```python
from build123d import *

# Parameters (mm, degrees)
SKETCH1_W               = 175
SKETCH1_H               = 260
BOSS_EXTRUDE1_DEPTH     = 3
SKETCH4_W               = 8.7
SKETCH4_H               = 8.7
BOSS_EXTRUDE3_DEPTH     = 328
MIRROR5_COPY_1_SKETCH_W = 8.7
MIRROR5_COPY_1_SKETCH_H = 8.7
MIRROR5_COPY_1_DEPTH    = 328
SKETCH6_W               = 38
SKETCH6_H               = 39
SKETCH6_W_2             = 34
SKETCH6_H_2             = 35
EXTRUDE_THIN1_DEPTH     = 10
SKETCH7_W               = 5.74
SKETCH7_H               = 5.74
BOSS_EXTRUDE5_DEPTH     = 8.5
SKETCH9_R               = 10.5
SKETCH9_R_2             = 6.5
EXTRUDE_THIN2_DEPTH     = 18
CUT_EXTRUDE1_DEPTH      = 367.180283467
CUT_EXTRUDE1_DEPTH_BACK = 367.180283467
SKETCH10_R              = 2.5
SKETCH11_R              = 2.5
BOSS_EXTRUDE6_DEPTH     = 3
CUT_EXTRUDE2_DEPTH      = 1
MIRROR7_COPY_1_SKETCH_R = 2.5
MIRROR7_COPY_1_DEPTH    = 3
MIRROR7_COPY_2_DEPTH    = 1


with BuildPart() as part:
    # Sketch1 → Boss-Extrude1 (new body)
    with BuildSketch(Plane(origin=(0, 0, 0), x_dir=(1, 0, 0), z_dir=(0, 1, 0))):
        Rectangle(SKETCH1_W, SKETCH1_H)
    extrude(amount=BOSS_EXTRUDE1_DEPTH)

    # Sketch4 → Boss-Extrude3 (add)
    with BuildSketch(Plane.XZ):
        with Locations((81.15, -123.65)):
            Rectangle(SKETCH4_W, SKETCH4_H)
    boss_extrude3 = extrude(amount=BOSS_EXTRUDE3_DEPTH)

    # Mirror3: Boss-Extrude3 across plane
    add(boss_extrude3.mirror(Plane.XY))

    # Mirror5: Boss-Extrude3 across plane
    add(boss_extrude3.mirror(Plane(origin=(0, 0, 0), x_dir=(0, 0, 1), z_dir=(1, 0, 0))))

    # Mirror5 copy 1 sketch → Mirror5 copy 1 (add)
    with BuildSketch(Plane(origin=(0, 0, 0), x_dir=(-1, 0, 0), z_dir=(0, -1, 0))):
        with Locations((81.15, -123.65)):
            Rectangle(MIRROR5_COPY_1_SKETCH_W, MIRROR5_COPY_1_SKETCH_H)
    extrude(amount=MIRROR5_COPY_1_DEPTH)

    # Sketch6 → Extrude-Thin1 (add)
    with BuildSketch(Plane(origin=(0, 0, -130), x_dir=(-1, 0, 0), z_dir=(0, 0, -1))):
        with Locations((0, -19.5)):
            Rectangle(SKETCH6_W, SKETCH6_H)
        with Locations((0, -19.5)):
            Rectangle(SKETCH6_W_2, SKETCH6_H_2, mode=Mode.SUBTRACT)
    extrude(amount=-EXTRUDE_THIN1_DEPTH)

    # Sketch7 → Boss-Extrude5 (add)
    with BuildSketch(Plane.XY.offset(-120)):
        with Locations((14.13, -4.87)):
            Rectangle(SKETCH7_W, SKETCH7_H)
        with Locations((-14.13, -4.87)):
            Rectangle(SKETCH7_W, SKETCH7_H)
        with Locations((-14.13, -34.13)):
            Rectangle(SKETCH7_W, SKETCH7_H)
        with Locations((14.13, -34.13)):
            Rectangle(SKETCH7_W, SKETCH7_H)
    extrude(amount=-BOSS_EXTRUDE5_DEPTH)

    # Sketch9 → Extrude-Thin2 (add)
    with BuildSketch(Plane.XZ):
        Circle(SKETCH9_R)
        Circle(SKETCH9_R_2, mode=Mode.SUBTRACT)
    extrude(amount=EXTRUDE_THIN2_DEPTH)

    # Sketch10 → Cut-Extrude1 (cut, two sides: drawn at the far end of the back side and taken through both)
    with BuildSketch(Plane(origin=(10.5, 0, 0), x_dir=(0, 0, -1), z_dir=(1, 0, 0)).offset(-CUT_EXTRUDE1_DEPTH_BACK)):
        with Locations((0, -10)):
            Circle(SKETCH10_R)
    extrude(amount=CUT_EXTRUDE1_DEPTH + CUT_EXTRUDE1_DEPTH_BACK, mode=Mode.SUBTRACT)

    # Sketch11 → Boss-Extrude6 (add)
    with BuildSketch(Plane.XZ):
        with Locations(Location((-72.5, 80, 0), (0, 0, 90))):
            Circle(SKETCH11_R)
    boss_extrude6 = extrude(amount=BOSS_EXTRUDE6_DEPTH)

    # Sketch12 → Cut-Extrude2 (cut)
    with BuildSketch(Plane.XZ.offset(3)):
        Polygon((-70.5, 80), (-71.5, 81.732050808), (-73.5, 81.732050808), (-74.5, 80), (-73.5, 78.267949192), (-71.5, 78.267949192), align=None)
    cut_extrude2 = extrude(amount=-CUT_EXTRUDE2_DEPTH, mode=Mode.SUBTRACT)

    # Mirror6: Boss-Extrude6, Cut-Extrude2 across plane
    add(boss_extrude6.mirror(Plane(origin=(0, 0, 0), x_dir=(0, 0, 1), z_dir=(1, 0, 0))))
    add(cut_extrude2.mirror(Plane(origin=(0, 0, 0), x_dir=(0, 0, 1), z_dir=(1, 0, 0))), mode=Mode.SUBTRACT)

    # Mirror7: Boss-Extrude6, Cut-Extrude2 across plane
    add(boss_extrude6.mirror(Plane.XY))
    add(cut_extrude2.mirror(Plane.XY), mode=Mode.SUBTRACT)

    # Mirror7 copy 1 sketch → Mirror7 copy 1 (add)
    with BuildSketch(Plane(origin=(0, 0, 0), x_dir=(-1, 0, 0), z_dir=(0, -1, 0))):
        with Locations(Location((-72.5, 80, 0), (0, 0, 90))):
            Circle(MIRROR7_COPY_1_SKETCH_R)
    extrude(amount=MIRROR7_COPY_1_DEPTH)

    # Mirror7 copy 2 sketch → Mirror7 copy 2 (cut)
    with BuildSketch(Plane(origin=(0, -3, 0), x_dir=(-1, 0, 0), z_dir=(0, -1, 0))):
        Polygon((-70.5, 80), (-71.5, 81.732050808), (-73.5, 81.732050808), (-74.5, 80), (-73.5, 78.267949192), (-71.5, 78.267949192), align=None)
    extrude(amount=-MIRROR7_COPY_2_DEPTH, mode=Mode.SUBTRACT)


solid = part.part
```
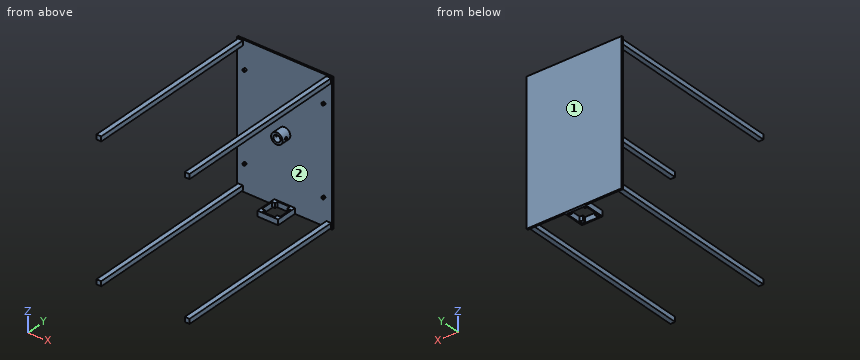
For this review, take the finished solid that the model builds, in its own axes (mm). Face numbers are marked on the shaded views. Give positions to 0.01 mm unless a question says otherwise; leave off trailing zeros. Order: outer loops, then holes, each group sorted by start corner. A loop starts at its lowest first (then second) coordinate and runs counter-clockwise, first axis right, second up.
1) Take a section at A-A (x = 0). Give the boundary of the cut face in (y, z), then the cut area to 3 significant figures.
2) Wall thickness on line 1 (Y direction, x = 7.2, z = 0); line 2 (Z direction, x = 0, y = -7.75); line 3 (Z direction, x = -8.6, y = -10): over which ranges is each line inside the solid? List them lowest first.
3) Take a section at C-C (z = 25.5). Give the boundary of the cut face in (x, y).
4) Take a section at D-D (x = 58). Give the boundary of the cut face in (y, z), then the cut area to 3 significant figures.
5) Take a section at B-B (y = -140). Give the boundary of the cut face in (x, z).
6) The part is to be moulded in two halves that separate along Z. For the marked faces 1 and 2, say which applies: released by +Z, released by -Z, zero draft, split by the parting line, or undercut.
7) Insertion check: pin 1 (7 mm diameter, centred on x = 81.5, y = -141, fed in from -Z); pin 2 (3 mm diameter, centred on y = -5, z = -126.5, fed in from +X); pin 3 (8 mm diameter, centred on x = 6.5, y = -45.5, fed in from +Z); pin 4 (0.8 mm diameter, centred on x = 72, y = -2.5, fed in from -Z). Each pin has a flat end and moves straight along its axis. Give the tip position at first contact, or say it passes through.
Derived:
1. outline: (-39, -130) - (-37, -130) - (-37, -120) - (-39, -120) - close; (-18, -10.5) - (0, -10.5) - (0, -120) - (-2, -120) - (-2, -130) - (3, -130) - (3, 130) - (0, 130) - (0, 10.5) - (-18, 10.5) - (-18, 6.5) - (0, 6.5) - (0, -6.5) - (-18, -6.5) - close
1. area: 964 mm2
2. line 1: y = -18 to -12.5, -7.5 to 3
2. line 2: z = -10.5 to -6.5, 6.5 to 10.5
2. line 3: z = -6.02 to -2.5, 2.5 to 6.02
3. outline: (-87.5, 0) - (87.5, 0) - (87.5, 3) - (-87.5, 3) - close
4. outline: (0, -130) - (3, -130) - (3, 130) - (0, 130) - close
4. area: 780 mm2
5. outline: (-85.5, -128) - (-76.8, -128) - (-76.8, -119.3) - (-85.5, -119.3) - close; (-85.5, 119.3) - (-76.8, 119.3) - (-76.8, 128) - (-85.5, 128) - close; (76.8, -128) - (85.5, -128) - (85.5, -119.3) - (76.8, -119.3) - close; (76.8, 119.3) - (85.5, 119.3) - (85.5, 128) - (76.8, 128) - close
6. face 1: zero draft
6. face 2: undercut
7. pin 1: stops at z = -128
7. pin 2: stops at x = 85.5
7. pin 3: passes through
7. pin 4: stops at z = -82.5
